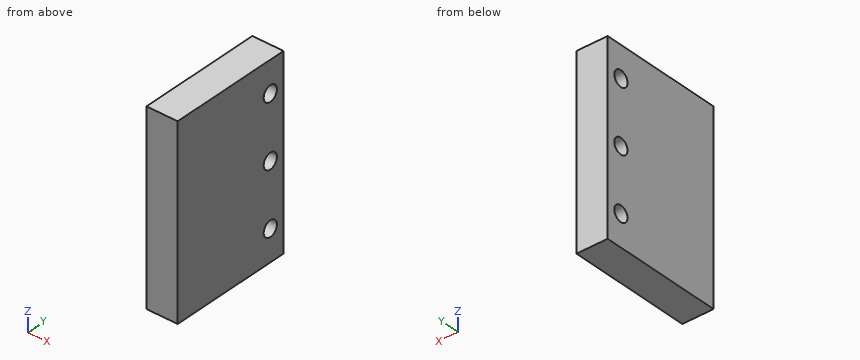
from build123d import *

# Parameters (mm, degrees)
BOSS_EXTRUDE1_DEPTH      = 38.1
F_1_4_20_THREADED_HOLE_D = 6.35


with BuildPart() as part:
    # Sketch2 → Boss-Extrude1 (new, symmetric)
    with BuildSketch(Plane.XY):
        Polygon((-6.35, 25.4), (6.35, 25.4), (6.35, -12.7), (6.35, -25.4), (-6.35, -25.4), (-6.35, 12.7), align=None)
    extrude(amount=BOSS_EXTRUDE1_DEPTH, both=True)

    # 1/4"-20 threaded hole (through all)
    with Locations(Plane(origin=(6.35, 0, 0), x_dir=(0, 0, -1), z_dir=(1, 0, 0))):
        with Locations((-25.4, 19.05), (0, 19.05), (25.4, 19.05)):
            Hole(F_1_4_20_THREADED_HOLE_D / 2)


solid = part.part
Design review of the part built by this model. Coordinates are the model's own, in mm. Coordinates: 2 decimals unless noted, no trailing zeros. Loops run counter-clockwise (first coordinate to the right, second up) from the corner with the lowest first, then second, coordinate; pieces in that order, holes last. Notation, with made-up numbers: (60, 64.25) - (69, 64.25) arc R7 ccw to (69, 71.25) - close; hole circle Ø1 at (49, 69). An arc over 180 degrees is marked (long way). Use CSV: the item, a comma, the result in double quotes. Start each with the question number.
1. Add section D-D on z = 2. Give the boundary of the cut face in (x, y), plus the area to 3 significant figures.
2. To check wall thickness, follow probe 1 along Y at (x, z) = (-3.5, 25.4) (3 decimals); probe 2 along Y at (x, z) = (5.5, 27). State the ranges of each line that lie inside material, in increasing order.
3. Add section B-B on x = 1.75. Give the boundary of the cut face in (y, z) (3 decimals), plus the area to 3 significant figures.
4. Add section A-A on z = -25.4. Give the boundary of the cut face in (x, y) (3 decimals), plus the area to 3 significant figures.
5. Add section C-C on y = 19.05. Give the boundary of the cut face in (x, z) (3 decimals).
Resolved:
1,outline,"(-6.35, -25.4) - (6.35, -25.4) - (6.35, 16.58) - (-6.35, 16.58) - close; (-6.35, 21.52) - (6.35, 21.52) - (6.35, 25.4) - (-6.35, 25.4) - close"
1,area,"583 mm2"
2,probe 1,"-25.4 to 15.875, 22.225 to 25.4"
2,probe 2,"-25.4 to 16.31, 21.79 to 25.4"
3,outline,"(-25.4, -38.1) - (25.4, -38.1) - (25.4, 38.1) - (-25.4, 38.1) - close; hole circle Ø6.35 at (19.05, -25.4); hole circle Ø6.35 at (19.05, 0); hole circle Ø6.35 at (19.05, 25.4)"
3,area,"3,780 mm2"
4,outline,"(-6.35, -25.4) - (6.35, -25.4) - (6.35, 15.875) - (-6.35, 15.875) - close; (-6.35, 22.225) - (6.35, 22.225) - (6.35, 25.4) - (-6.35, 25.4) - close"
4,area,"565 mm2"
5,outline,"(-6.35, -38.1) - (6.35, -38.1) - (6.35, -28.575) - (-6.35, -28.575) - close; (-6.35, -22.225) - (6.35, -22.225) - (6.35, -3.175) - (-6.35, -3.175) - close; (-6.35, 3.175) - (6.35, 3.175) - (6.35, 22.225) - (-6.35, 22.225) - close; (-6.35, 28.575) - (6.35, 28.575) - (6.35, 38.1) - (-6.35, 38.1) - close"
